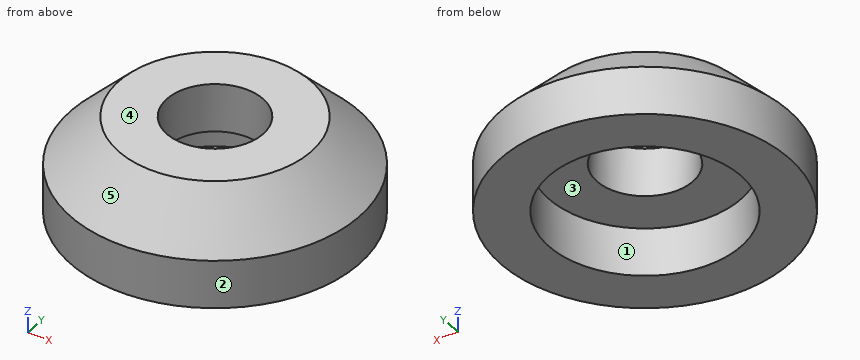
```python
from build123d import *

# Parameters (mm, degrees)
SKETCH1_R           = 7.5
SKETCH1_R_2         = 2.5
BOSS_EXTRUDE1_DEPTH = 5
CHAMFER1_SIZE       = 2.5
SKETCH2_R           = 5
CUT_EXTRUDE1_DEPTH  = 2.5


with BuildPart() as part:
    # Sketch1 → Boss-Extrude1 (new body)
    with BuildSketch(Plane.XY):
        Circle(SKETCH1_R)
        Circle(SKETCH1_R_2, mode=Mode.SUBTRACT)
    extrude(amount=BOSS_EXTRUDE1_DEPTH)

    # Chamfer1
    chamfer1_edges = [part.edges().sort_by_distance(p)[0] for p in [
        (-7.5, 0, 5),
    ]]
    chamfer(chamfer1_edges, length=CHAMFER1_SIZE)

    # Sketch2 → Cut-Extrude1 (cut)
    with BuildSketch(Plane(origin=(0, 0, 0), x_dir=(-1, 0, 0), z_dir=(0, 0, -1))):
        Circle(SKETCH2_R)
    extrude(amount=-CUT_EXTRUDE1_DEPTH, mode=Mode.SUBTRACT)


solid = part.part
```
The listing builds one solid part. Answer for the finished solid, in the listing's coordinates (mm). Face numbers are marked on the shaded views. A direction names the side the tool comes from. Coordinates: 2 decimals unless noted, no trailing zeros. Write each loop counter-clockwise with the first axis right and the second up, starting at its lowest first coordinate (ties: lowest second). Pieces come first, ordered by that corner, then holes. Notation, with made-up numbers: (59, -40) - (97, -40) arc R18 cw to (97, -11) - close; hole circle Ø6 at (62, -26). An arc over 180 degrees is marked (long way). Return JSON: item names as keys, results as strings. Group by question number.
1. Straight lines are drawn through the part: L1, parallel to Z at x = -3, y = -3; L2, parallel to Y at x = 0, z = 1.7; L3, parallel to Y at x = -2.25, z = 4. For each, find the intervals that lie inside material, in ascending order.
2. Given pin 1 (1.5 mm diameter, centred on x = -1.5, z = 3, fed in from +Y); pin 2 (8 mm diameter, centred on x = 0, y = 0, fed in from +Z); pin 3 (1.5 mm diameter, centred on y = 2, z = 1.5, fed in from -X), each flat-ended and moving along its own axis, determine where each tip first touches the part or whether it passes through.
3. A cutting plane is placed at A-A, the plane x = 0. Determine the outline of the cut face in (y, z).
4. A cutting plane is placed at B-B, the plane z = 3.55. Determine the outline of the cut face in (x, y), plus the area to 3 significant figures.
5. A cutting plane is placed at C-C, the plane z = 4.55. Determine the outline of the cut face in (x, y), plus the area to 3 significant figures.
6. Determine the mould class of the marked faces 3, 4 and 5 for opening direction X: released by +X, released by -X, zero draft, split by the parting line, or undercut.
7. Which of the six approach directions +Z, -Z, +X, -X, +Y, -Y give full straight-line access (tool end or side, diameter ignored) to the marked faces 1 and 2?
Ans:
{
 "1": {"L1": "2.5 to 5", "L2": "-7.5 to -5, 5 to 7.5", "L3": "-5.56 to -1.09, 1.09 to 5.56"},
 "2": {"pin 1": "y = 7.44", "pin 2": "z = 5", "pin 3": "x = -7.4"},
 "3": {"outline": "(-7.5, 0) - (-5, 0) - (-5, 2.5) - (-2.5, 2.5) - (-2.5, 5) - (-5, 5) - (-7.5, 2.5) - close; (2.5, 2.5) - (5, 2.5) - (5, 0) - (7.5, 0) - (7.5, 2.5) - (5, 5) - (2.5, 5) - close"},
 "4": {"outline": "circle Ø12.9 at (0, 0); hole circle Ø5 at (0, 0)", "area": "111 mm²"},
 "5": {"outline": "circle Ø10.9 at (0, 0); hole circle Ø5 at (0, 0)", "area": "73.7 mm²"},
 "6": {"face 3": "undercut", "face 4": "zero draft", "face 5": "split by the parting line"},
 "7": {"face 1": "-Z", "face 2": "+Z, -Z"}
}
